Model file for the job. Use its own axes, mm. Give positions to 0.01 mm unless a question says otherwise; leave off trailing zeros. Order: outer loops, then holes, each group sorted by start corner. A loop starts at its lowest first (then second) coordinate and runs counter-clockwise, first axis right, second up. Notation, with made-up numbers: (83.25, 37.5) -> (131.25, 37.5) arc R22 ccw to (131.25, 44.5) -> close; hole circle Ø3 at (75.25, 72.5). An arc over 180 degrees is marked (long way). Use CSV: the item, a comma, the result in double quotes. Start each with the question number.
1. Drop flat-ended pins along their axis: pin 1 (1 mm diameter, centred on x = 84.5, z = -139.5, fed in from -Y); pin 2 (1.5 mm diameter, centred on y = 203.5, z = -146.5, fed in from +X); pin 3 (0.9 mm diameter, centred on y = 207, z = -82.5, fed in from -X). Give the stop position or say it passes through.
2. Wall check: line 1 (X direction, y = 200.25, z = -277); line 2 (Y direction, x = 99, z = -170); line 3 (X direction, y = 206.5, z = -209.5). Give the ranges that are in metal, low to high. Write a range as from..to.
3. Pull direction X, two halves, no side cores. Call faces 1 (the cylindrical face through (124.196, 206.239, -151.913)), 2 (the cylindrical face through (43.76, 206.43, -134.34)): released by +X, released by -X, zero draft, split by the parting line, or undercut.
4. Cut at C-C on z = -70.8. List the corners of the cut face in (x, y), then the cut area to 3 significant figures.
5. Cut at A-A on z = -239. List the corners of the cut face in (x, y).
6. Cut at D-D on y = 198. List the corners of the cut face in (x, z).
7. Cut at B-B on z = -150.8. List the corners of the cut face in (x, y).
```python
from build123d import *

# Parameters (mm, degrees)
SKETCH1_W                   = 90
SKETCH1_H                   = 290
BASE_FLANGE1_DEPTH          = 3
SM_EDGE_FLANGE_1_DEPTH      = 290
SM_EDGE_FLANGE_1_BEND_DEPTH = 290
INDENT1_START               = 23
INDENT1_DEPTH               = 104
INDENT1_START_2             = 26.270388893
INDENT1_2_DEPTH             = 97.459222009
INDENT1_3_DEPTH             = 0.729611107
INDENT1_START_3             = 123
INDENT1_4_DEPTH             = 0.729610902
INDENT1_START_4             = 119.9999999
INDENT1_5_DEPTH             = 6.0000001
INDENT1_START_5             = 24
INDENT1_6_DEPTH             = 6
INDENT1_START_6             = -290
INDENT1_7_DEPTH             = 6.65
INDENT2_START               = 23
INDENT2_DEPTH               = 104
INDENT2_START_2             = -11.0000001
INDENT2_2_DEPTH             = 11.0000001
INDENT2_START_3             = 24
INDENT2_3_DEPTH             = 102
CUT_EXTRUDE1_DEPTH          = 317.754179273
CUT_EXTRUDE1_DEPTH_BACK     = 317.754179273
SKETCH15_R                  = 4.2
CUT_EXTRUDE2_DEPTH          = 317.754179273
CUT_EXTRUDE2_DEPTH_BACK     = 317.754179273


with BuildPart() as part:
    # Base-Flange1: sheet metal written as solids
    # Sketch1 → Base-Flange1 (new body)
    with BuildSketch(Plane(origin=(0, 207.95, 0), x_dir=(1, 0, 0), z_dir=(0, 1, 0))):
        with Locations((75, 145)):
            Rectangle(SKETCH1_W, SKETCH1_H)
    extrude(amount=-BASE_FLANGE1_DEPTH)

    # 邊線-凸緣1: sheet metal written as solids
    # 邊線-凸緣1 section (on a plane across the edge) → 邊線-凸緣1 (add)
    with BuildSketch(Plane(origin=(27, 204.95, 0), x_dir=(1, 0, 0), z_dir=(0, 0, -1))):
        with BuildLine():
            Line((-3, 3), (-3, 15.9))
            Line((-3, 15.9), (0, 15.9))
            Line((0, 15.9), (0, 3))
            ThreePointArc((0, 3), (0.878679656, 0.878679656), (3, 0))
            Line((3, 0), (3, -3))
            ThreePointArc((3, -3), (-1.242640687, -1.242640687), (-3, 3))
        make_face()
    extrude(amount=SM_EDGE_FLANGE_1_DEPTH)

    # 邊線-凸緣1 section 2 (on a plane across the edge) → 邊線-凸緣1 bend (add)
    with BuildSketch(Plane(origin=(123, 204.95, -290), x_dir=(-1, 0, 0), z_dir=(0, 0, 1))):
        with BuildLine():
            Line((-3, 3), (-3, 15.9))
            Line((-3, 15.9), (0, 15.9))
            Line((0, 15.9), (0, 3))
            ThreePointArc((0, 3), (0.878679656, 0.878679656), (3, 0))
            Line((3, 0), (3, -3))
            ThreePointArc((3, -3), (-1.242640687, -1.242640687), (-3, 3))
        make_face()
    extrude(amount=SM_EDGE_FLANGE_1_BEND_DEPTH)

    # Indent1: read off the stored shape, not the designer's step
    # Indent1 outline → Indent1 (cut)
    with BuildSketch(Plane.YZ.offset(INDENT1_START)):
        with BuildLine():
            Line((192.05, -290), (207.95, -290))
            ThreePointArc((207.95, -290), (200, -282.05), (192.05, -290))
        make_face()
    extrude(amount=INDENT1_DEPTH, mode=Mode.SUBTRACT)

    # Indent2: read off the stored shape, not the designer's step
    # Indent2 outline → Indent2 (cut)
    with BuildSketch(Plane.YZ.offset(INDENT2_START)):
        with BuildLine():
            ThreePointArc((189.05, -6.433311744), (197.7062633, -12.491147744), (207.950014124, -9.903902031))
            Line((207.950014124, -9.903902031), (209, -9.061062257))
            Line((209, -9.061062257), (209, 1))
            Line((209, 1), (188, 1))
            Line((188, 1), (188, 0))
            Line((188, 0), (188, -4.64612958))
            Line((188, -4.64612958), (189.05, -6.433311744))
        make_face()
    extrude(amount=INDENT2_DEPTH, mode=Mode.SUBTRACT)

    # Sketch15 → Cut-Extrude1 (cut, two sides: drawn at the far end of the back side and taken through both)
    with BuildSketch(Plane(origin=(0, 207.95, 0), x_dir=(1, 0, 0), z_dir=(0, 1, 0)).offset(-CUT_EXTRUDE1_DEPTH_BACK)):
        with Locations((41.5, 270.8)):
            Circle(SKETCH15_R)
        with Locations((108.5, 270.8)):
            Circle(SKETCH15_R)
        with Locations((41.5, 250.8)):
            Circle(SKETCH15_R)
        with Locations((108.5, 250.8)):
            Circle(SKETCH15_R)
        with Locations((41.5, 230.8)):
            Circle(SKETCH15_R)
        with Locations((108.5, 230.8)):
            Circle(SKETCH15_R)
        with Locations((41.5, 210.8)):
            Circle(SKETCH15_R)
        with Locations((108.5, 210.8)):
            Circle(SKETCH15_R)
        with Locations((41.5, 190.8)):
            Circle(SKETCH15_R)
        with Locations((108.5, 190.8)):
            Circle(SKETCH15_R)
        with Locations((41.5, 170.8)):
            Circle(SKETCH15_R)
        with Locations((108.5, 170.8)):
            Circle(SKETCH15_R)
        with Locations((41.5, 150.8)):
            Circle(SKETCH15_R)
        with Locations((108.5, 150.8)):
            Circle(SKETCH15_R)
        with Locations((41.5, 130.8)):
            Circle(SKETCH15_R)
        with Locations((108.5, 130.8)):
            Circle(SKETCH15_R)
        with Locations((41.5, 110.8)):
            Circle(SKETCH15_R)
        with Locations((108.5, 110.8)):
            Circle(SKETCH15_R)
        with Locations((41.5, 90.8)):
            Circle(SKETCH15_R)
        with Locations((108.5, 90.8)):
            Circle(SKETCH15_R)
        with Locations((41.5, 70.8)):
            Circle(SKETCH15_R)
        with Locations((108.5, 70.8)):
            Circle(SKETCH15_R)
    extrude(amount=CUT_EXTRUDE1_DEPTH + CUT_EXTRUDE1_DEPTH_BACK, mode=Mode.SUBTRACT)

    # Sketch16 → Cut-Extrude2 (cut, two sides: drawn at the far end of the back side and taken through both)
    with BuildSketch(Plane(origin=(0, 207.95, 0), x_dir=(1, 0, 0), z_dir=(0, 1, 0)).offset(-CUT_EXTRUDE2_DEPTH_BACK)):
        with BuildLine():
            Line((55, 54.903913368), (55, 119.903913368))
            ThreePointArc((55, 119.903913368), (75, 139.903913368), (95, 119.903913368))
            Line((95, 119.903913368), (95, 54.903913368))
            ThreePointArc((95, 54.903913368), (75, 34.903913368), (55, 54.903913368))
        make_face()
        with BuildLine():
            Line((55, 180), (55, 245))
            ThreePointArc((55, 245), (75, 265), (95, 245))
            Line((95, 245), (95, 180))
            ThreePointArc((95, 180), (75, 160), (55, 180))
        make_face()
    extrude(amount=CUT_EXTRUDE2_DEPTH + CUT_EXTRUDE2_DEPTH_BACK, mode=Mode.SUBTRACT)


with BuildPart() as body_2:
    # Indent1 2 outline → Indent1 2 (new body)
    with BuildSketch(Plane.YZ.offset(INDENT1_START_2)):
        with BuildLine():
            Line((204.95, -285.559279338), (204.95, -290))
            Line((204.95, -290), (206.65, -290))
            ThreePointArc((206.65, -290), (206.210475022, -287.622501314), (204.95, -285.559279338))
        make_face()
    extrude(amount=INDENT1_2_DEPTH)

    # Indent1 3 outline → Indent1 3 (add)
    with BuildSketch(Plane.YZ.offset(INDENT1_START_2)):
        with BuildLine():
            Line((193.35, -290), (204.95, -290))
            Line((204.95, -290), (204.95, -285.559279338))
            ThreePointArc((204.95, -285.559279338), (197.622501314, -283.789524978), (193.35, -290))
        make_face()
    extrude(amount=INDENT1_3_DEPTH)

    # Indent1 4 outline → Indent1 4 (add)
    with BuildSketch(Plane.YZ.offset(INDENT1_START_3)):
        with BuildLine():
            Line((193.35, -290), (204.95, -290))
            Line((204.95, -290), (204.95, -285.559279338))
            ThreePointArc((204.95, -285.559279338), (197.622501314, -283.789524978), (193.35, -290))
        make_face()
    extrude(amount=INDENT1_4_DEPTH)

    # Indent1 5 outline → Indent1 5 (add)
    with BuildSketch(Plane.YZ.offset(INDENT1_START_4)):
        with BuildLine():
            Line((193.35, -290), (206.65, -290))
            ThreePointArc((206.65, -290), (200, -283.35), (193.35, -290))
        make_face()
    extrude(amount=INDENT1_5_DEPTH)

    # Indent1 6 outline → Indent1 6 (add)
    with BuildSketch(Plane.YZ.offset(INDENT1_START_5)):
        with BuildLine():
            Line((193.35, -290), (206.65, -290))
            ThreePointArc((206.65, -290), (200, -283.35), (193.35, -290))
        make_face()
    extrude(amount=INDENT1_6_DEPTH)

    # Indent1 7 outline → Indent1 7 (cut)
    with BuildSketch(Plane.XY.offset(INDENT1_START_6)):
        with BuildLine():
            Line((123, 192), (123, 201.95))
            ThreePointArc((123, 201.95), (122.121320344, 204.071320344), (120, 204.95))
            Line((120, 204.95), (119.9999999, 192))
            Line((119.9999999, 192), (123, 192))
        make_face()
        with BuildLine():
            Line((27, 192), (30, 192))
            Line((30, 192), (30, 204.95))
            ThreePointArc((30, 204.95), (27.878679656, 204.071320344), (27, 201.95))
            Line((27, 201.95), (27, 192))
        make_face()
        with BuildLine():
            ThreePointArc((123.729603466, 206.650006169), (125.402666971, 204.559825589), (126, 201.95))
            Line((126, 201.95), (126, 208))
            Line((126, 208), (122.028355761, 208))
            Line((122.028355761, 208), (123.729603466, 206.650006169))
        make_face()
        with BuildLine():
            Line((24, 208), (24, 201.95))
            ThreePointArc((24, 201.95), (24.597331636, 204.559822705), (26.270391517, 206.650002187))
            Line((26.270391517, 206.650002187), (27.971640511, 208))
            Line((27.971640511, 208), (24, 208))
        make_face()
    extrude(amount=INDENT1_7_DEPTH, mode=Mode.SUBTRACT)


with BuildPart() as body_3:
    # Indent2 2 outline → Indent2 2 (new body)
    with BuildSketch(Plane.XY.offset(INDENT2_START_2)):
        with BuildLine():
            Line((24, 201.95), (24, 189.05))
            Line((24, 189.05), (27, 189.05))
            Line((27, 189.05), (27, 201.95))
            ThreePointArc((27, 201.95), (27.878679656, 204.071320344), (30, 204.95))
            Line((30, 204.95), (120, 204.95))
            ThreePointArc((120, 204.95), (122.121320344, 204.071320344), (123, 201.95))
            Line((123, 201.95), (123, 189.05))
            Line((123, 189.05), (126, 189.05))
            Line((126, 189.05), (126, 201.95))
            ThreePointArc((126, 201.95), (124.242640687, 206.192640687), (120, 207.95))
            Line((120, 207.95), (30, 207.95))
            ThreePointArc((30, 207.95), (25.757359313, 206.192640687), (24, 201.95))
        make_face()
    extrude(amount=INDENT2_2_DEPTH)

    # Indent2 3 outline → Indent2 3 (cut)
    with BuildSketch(Plane.YZ.offset(INDENT2_START_3)):
        with BuildLine():
            Line((207.95, -11.0000001), (207.950016725, -7.602449216))
            ThreePointArc((207.950016725, -7.602449216), (204.322791843, -10.115012145), (200.000000001, -11))
            Line((200.000000001, -11), (207.95, -11.0000001))
        make_face()
        with BuildLine():
            Line((189.05, -11.0000001), (200.000000001, -11))
            ThreePointArc((200.000000001, -11), (192.601479194, -8.140140655), (189.05, -1.047616342))
            Line((189.05, -1.047616342), (189.05, -11.0000001))
        make_face()
    extrude(amount=INDENT2_3_DEPTH, mode=Mode.SUBTRACT)


solid = part.part
```
Verdict:
1,pin 1,"y = 204.95"
1,pin 2,"x = 125.95"
1,pin 3,"x = 26.15"
2,line 1,"24..27, 123..126"
2,line 2,"204.95..207.95"
2,line 3,"26.09..37.51, 45.49..55, 95..104.51, 112.49..123.91"
3,face 1,"released by +X"
3,face 2,"undercut"
4,outline,"(24, 189.05) -> (27, 189.05) -> (27, 201.95) arc R3 cw to (30, 204.95) -> (37.3, 204.95) -> (37.3, 207.95) -> (30, 207.95) arc R6 ccw to (24, 201.95) -> close; (45.7, 204.95) -> (55, 204.95) -> (55, 207.95) -> (45.7, 207.95) -> close; (95, 204.95) -> (104.3, 204.95) -> (104.3, 207.95) -> (95, 207.95) -> close; (112.7, 204.95) -> (120, 204.95) arc R3 cw to (123, 201.95) -> (123, 189.05) -> (126, 189.05) -> (126, 201.95) arc R6 ccw to (120, 207.95) -> (112.7, 207.95) -> close"
4,area,"219 mm^2"
5,outline,"(24, 189.05) -> (27, 189.05) -> (27, 201.95) arc R3 cw to (30, 204.95) -> (55, 204.95) -> (55, 207.95) -> (30, 207.95) arc R6 ccw to (24, 201.95) -> close; (95, 204.95) -> (120, 204.95) arc R3 cw to (123, 201.95) -> (123, 189.05) -> (126, 189.05) -> (126, 201.95) arc R6 ccw to (120, 207.95) -> (95, 207.95) -> close"
6,outline,"(24, -282.31) -> (27, -282.31) -> (27, -12.54) -> (24, -12.54) -> close; (123, -282.31) -> (126, -282.31) -> (126, -12.54) -> (123, -12.54) -> close"
7,outline,"(24, 189.05) -> (27, 189.05) -> (27, 201.95) arc R3 cw to (30, 204.95) -> (37.3, 204.95) -> (37.3, 207.95) -> (30, 207.95) arc R6 ccw to (24, 201.95) -> close; (45.7, 204.95) -> (104.3, 204.95) -> (104.3, 207.95) -> (45.7, 207.95) -> close; (112.7, 204.95) -> (120, 204.95) arc R3 cw to (123, 201.95) -> (123, 189.05) -> (126, 189.05) -> (126, 201.95) arc R6 ccw to (120, 207.95) -> (112.7, 207.95) -> close"
